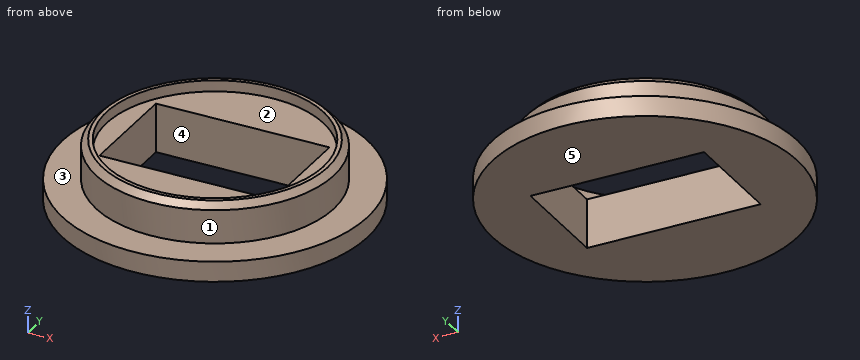
```python
from build123d import *

# Parameters (mm, degrees)
F0_R     = 19.05
F1_DEPTH = 2.54
F2_R     = 14.85
F3_DEPTH = 5
F4_W     = 21.7
F4_H     = 13.5
F5_DEPTH = 10
F6_R     = 13.55
F7_DEPTH = 1.4
F8_SIZE  = 0.8


with BuildPart() as f1:
    # F0 (on Top) → F1 (new body)
    with BuildSketch(Plane.XY):
        Circle(F0_R)
    extrude(amount=F1_DEPTH)

    # F2 (on face) → F3 (join)
    with BuildSketch(Plane.XY.offset(2.54)):
        Circle(F2_R)
    extrude(amount=F3_DEPTH)

    # F4 (on face) → F5 (cut)
    with BuildSketch(Plane.XY.offset(7.54)):
        with Locations((0.067133, -0.25862)):
            Rectangle(F4_W, F4_H)
    extrude(amount=-F5_DEPTH, mode=Mode.SUBTRACT)

    # F6 (on face) → F7 (cut)
    with BuildSketch(Plane.XY.offset(7.54)):
        Circle(F6_R)
    extrude(amount=-F7_DEPTH, mode=Mode.SUBTRACT)

    # F8
    f8_edges = [f1.edges().sort_by_distance(p)[0] for p in [
        (-14.85, 0, 7.54),
    ]]
    chamfer(f8_edges, length=F8_SIZE)


solid = f1.part
```
Source: CAD feature listing. Evaluate the final solid. Frame: model axes, mm. Face numbers are marked on the shaded views. A direction names the side the tool comes from. Round coordinates to 2 decimals unless told otherwise and drop trailing zeros. Write each loop counter-clockwise with the first axis right and the second up, starting at its lowest first coordinate (ties: lowest second). Pieces come first, ordered by that corner, then holes. Notation, with made-up numbers: M -36,50.25 L -10,50.25 A16 cw -10,75.25 Z; hole C 51.5,53.5 d4. An arc over 180 degrees is marked long. Answer as a JSON object with one key per item and string values. Group by question number.
(1) Section query C-C on z = 1.75. Output: boundary loops of the cut face in (x, y).
(2) Ray query, line 1 (Y direction, x = -0.5, z = 2.5); line 2 (Y direction, x = 0, z = 6.5); line 3 (Z direction, x = 3.5, y = 9). Return the intervals inside material, ascending. Write a range as [from, to].
(3) Section query B-B on z = 4.25. Output: boundary loops of the cut face in (x, y).
(4) Reachability of the marked faces 4 and 5 from +Z, -Z, +X, -X, +Y, -Y: full face, straight path, thin tool, end or side. Return the list, or none.
(5) Section query D-D on y = 16.5. Output: boundary loops of the cut face in (x, z), then the cut area to 3 significant figures.
(6) Section query A-A on x = 0. Output: boundary loops of the cut face in (y, z).
(7) First-contact query: pin 1 (1 mm diameter, centred on x = -12.5, z = 3.5, fed in from +Y); pin 2 (6 mm diameter, centred on x = -13, y = 13, fed in from +Z); pin 3 (1.8 mm diameter, centred on x = -4.5, z = 4, fed in from -Y). Flat tips, straight axial feed; report the tip coordinate or a pass-through.
(8) Mould query, pull axis X, two halves, no side actions, for the marked faces 1, 2 and 3. Classes: +X half, -X half, draft (parallel to the pull), parting line (faces both ways), or undercut.
Computed values:
{
 "1": {"outline": "C 0,0 d38.1; hole M -10.78,-7.01 L 10.92,-7.01 L 10.92,6.49 L -10.78,6.49 Z"},
 "2": {"line 1": "[-19.04, -7.01], [6.49, 19.04]", "line 2": "[-14.85, -13.55], [13.55, 14.85]", "line 3": "[0, 6.14]"},
 "3": {"outline": "C 0,0 d29.7; hole M -10.78,-7.01 L 10.92,-7.01 L 10.92,6.49 L -10.78,6.49 Z"},
 "4": {"face 4": "+Z, -Z", "face 5": "-Z, +X, -X, +Y, -Y"},
 "5": {"outline": "M -9.52,0 L 9.52,0 L 9.52,2.54 L -9.52,2.54 Z", "area": "48.4 mm^2"},
 "6": {"outline": "M -19.05,0 L -7.01,0 L -7.01,6.14 L -13.55,6.14 L -13.55,7.54 L -14.05,7.54 L -14.85,6.74 L -14.85,2.54 L -19.05,2.54 Z; M 6.49,0 L 19.05,0 L 19.05,2.54 L 14.85,2.54 L 14.85,6.74 L 14.05,7.54 L 13.55,7.54 L 13.55,6.14 L 6.49,6.14 Z"},
 "7": {"pin 1": "y = 8.75", "pin 2": "z = 2.54", "pin 3": "y = -14.41"},
 "8": {"face 1": "parting line", "face 2": "undercut", "face 3": "draft"}
}
